```python
from build123d import *

# Parameters (mm, degrees)
F0_W         = 108.091738075
F0_H         = 57.078147307
F1_DEPTH     = 50
F2_T         = -2.5
F3_R         = 1
F4_T1_DEPTH  = 48
F4_T3_DEPTH  = 106.091738075
F4_T5_DEPTH  = 55.078147307
F4_S9_W      = 1
F4_S9_H      = 1
F4_T10_DEPTH = 1
F4_S15_W     = 1
F4_S15_H     = 1
F4_T16_DEPTH = 1
F4_T20_ANGLE = 90
F4_T22_ANGLE = 90
F4_T24_ANGLE = 90
F5_W         = 18.639581278
F5_H         = 12.6642128453
F6_DEPTH     = 25


# Not quite as in the source:
# - a fillet or chamfer that OpenCascade refuses, or shapes differently, is made with other operations: its cross-section is extruded or revolved along the edge and cut away or added


with BuildPart() as f1:
    # F0 (on Top) → F1 (new body)
    with BuildSketch(Plane.XY):
        with Locations((-7.7590625733, 5.3510768339)):
            Rectangle(F0_W, F0_H)
    extrude(amount=F1_DEPTH)

    # F2
    f2_openings = [f1.faces().sort_by_distance(p)[0] for p in [
        (-7.759063, 5.351077, 50),
    ]]
    offset(amount=F2_T, openings=f2_openings)

    # F3
    f3_edges = [f1.edges().sort_by_distance(p)[0] for p in [
        (-7.759063, -23.187997, 50),
        (-61.804932, -23.187997, 25),
        (-7.759063, -20.687997, 50),
        (-59.304932, 5.351077, 50),
        (-61.804932, 5.351077, 50),
        (-7.759063, -23.187997, 0),
        (46.286806, -23.187997, 25),
        (43.786806, 5.351077, 50),
        (46.286806, 5.351077, 50),
        (46.286806, 5.351077, 0),
    ]]
    fillet(f3_edges, radius=F3_R)

    # F4: fillet of radius 1 on 3 edges, made by hand

    # F4_s2 → F4_t1 (cut)
    with BuildSketch(Plane.XY.offset(1)):
        with BuildLine():
            ThreePointArc((45.2868064642, 33.8901504874), (45.9939132454, 33.5972572686), (46.2868064642, 32.8901504874))
            Line((46.2868064642, 32.8901504874), (46.2868064642, 33.8901504874))
            Line((46.2868064642, 33.8901504874), (45.2868064642, 33.8901504874))
        make_face()
        with BuildLine():
            ThreePointArc((-60.8049316108, 33.8901504874), (-61.512038392, 33.5972572686), (-61.8049316108, 32.8901504874))
            Line((-61.8049316108, 32.8901504874), (-61.8049316108, 33.8901504874))
            Line((-61.8049316108, 33.8901504874), (-60.8049316108, 33.8901504874))
        make_face()
    extrude(amount=F4_T1_DEPTH, mode=Mode.SUBTRACT)

    # F4_s4 → F4_t3 (cut)
    with BuildSketch(Plane.YZ.offset(-60.8049316108)):
        with BuildLine():
            ThreePointArc((33.8901504874, 49), (33.5972572686, 49.7071067812), (32.8901504874, 50))
            Line((32.8901504874, 50), (33.8901504874, 50))
            Line((33.8901504874, 50), (33.8901504874, 49))
        make_face()
        with BuildLine():
            ThreePointArc((33.8901504874, 1), (33.5972572686, 0.2928932188), (32.8901504874, 0))
            Line((32.8901504874, 0), (33.8901504874, 0))
            Line((33.8901504874, 0), (33.8901504874, 1))
        make_face()
    extrude(amount=F4_T3_DEPTH, mode=Mode.SUBTRACT)

    # F4_s6 → F4_t5 (cut)
    with BuildSketch(Plane.XZ.offset(-32.8901504874)):
        with BuildLine():
            ThreePointArc((-60.8049316108, 0), (-61.512038392, 0.2928932188), (-61.8049316108, 1))
            Line((-61.8049316108, 1), (-61.8049316108, 0))
            Line((-61.8049316108, 0), (-60.8049316108, 0))
        make_face()
    extrude(amount=F4_T5_DEPTH, mode=Mode.SUBTRACT)


with BuildPart() as f4_tool8:
    # F4_s9 → F4_t10 (new body)
    with BuildSketch(Plane.XY.offset(1)):
        with Locations((-61.3049316108, -22.6879968196)):
            Rectangle(F4_S9_W, F4_S9_H)
    extrude(amount=-F4_T10_DEPTH)

    # F4_s11 → F4_t12 (revolve, cut)
    with BuildSketch(Plane(origin=(-60.8049316108, -22.1879968196, 1), x_dir=(0.7071067812, 0.7071067812, 0), z_dir=(-0.7071067812, 0.7071067812, 0))):
        with BuildLine():
            ThreePointArc((0, -1), (1, 0), (0, 1))
            Line((0, 1), (0, -1))
        make_face()
    revolve(axis=Axis((-60.8049316108, -22.1879968196, 1), (0, 0, -1)), mode=Mode.SUBTRACT)


with BuildPart() as f1_1:
    add(f1.part)

    # F4_t7: cut F4_tool8
    add(f4_tool8.part, mode=Mode.SUBTRACT)


with BuildPart() as f4_tool14:
    # F4_s15 → F4_t16 (new body)
    with BuildSketch(Plane.XZ.offset(-32.8901504874)):
        with Locations((-61.3049316108, 0.5)):
            Rectangle(F4_S15_W, F4_S15_H)
    extrude(amount=-F4_T16_DEPTH)

    # F4_s17 → F4_t18 (revolve, cut)
    with BuildSketch(Plane(origin=(-60.8049316108, 32.8901504874, 1), x_dir=(0.7071067812, 0, 0.7071067812), z_dir=(-0.7071067812, 0, 0.7071067812))):
        with BuildLine():
            ThreePointArc((0, -1), (1, 0), (0, 1))
            Line((0, 1), (0, -1))
        make_face()
    revolve(axis=Axis((-60.8049316108, 32.8901504874, 1), (0, 1, 0)), mode=Mode.SUBTRACT)


with BuildPart() as f1_2:
    add(f1_1.part)

    # F4_t13: cut F4_tool14
    add(f4_tool14.part, mode=Mode.SUBTRACT)

    # F4_s19 → F4_t20 (revolve, cut)
    with BuildSketch(Plane.XY.offset(49)):
        with BuildLine():
            ThreePointArc((45.2868064642, 33.8901504874), (45.9939132454, 33.5972572686), (46.2868064642, 32.8901504874))
            Line((46.2868064642, 32.8901504874), (46.2868064642, 33.8901504874))
            Line((46.2868064642, 33.8901504874), (45.2868064642, 33.8901504874))
        make_face()
    revolve(axis=Axis((45.2868064642, 33.8901504874, 49), (0, -1, 0)), revolution_arc=F4_T20_ANGLE, mode=Mode.SUBTRACT)

    # F4_s21 → F4_t22 (revolve, cut)
    with BuildSketch(Plane.XY.offset(49)):
        with BuildLine():
            ThreePointArc((-60.8049316108, 33.8901504874), (-61.512038392, 33.5972572686), (-61.8049316108, 32.8901504874))
            Line((-61.8049316108, 32.8901504874), (-61.8049316108, 33.8901504874))
            Line((-61.8049316108, 33.8901504874), (-60.8049316108, 33.8901504874))
        make_face()
    revolve(axis=Axis((-60.8049316108, 33.8901504874, 49), (0, 1, 0)), revolution_arc=F4_T22_ANGLE, mode=Mode.SUBTRACT)

    # F4_s23 → F4_t24 (revolve, cut)
    with BuildSketch(Plane.XY.offset(1)):
        with BuildLine():
            ThreePointArc((45.2868064642, 33.8901504874), (45.9939132454, 33.5972572686), (46.2868064642, 32.8901504874))
            Line((46.2868064642, 32.8901504874), (46.2868064642, 33.8901504874))
            Line((46.2868064642, 33.8901504874), (45.2868064642, 33.8901504874))
        make_face()
    revolve(axis=Axis((45.2868064642, 33.8901504874, 1), (0, 1, 0)), revolution_arc=F4_T24_ANGLE, mode=Mode.SUBTRACT)

    # F5 (on face) → F6 (cut)
    with BuildSketch(Plane.YZ.offset(46.2868064642)):
        with Locations((9.319790639, 18.1044735946)):
            Rectangle(F5_W, F5_H)
    extrude(amount=-F6_DEPTH, mode=Mode.SUBTRACT)


solid = f1_2.part
```
Work out the finished part from the listing and answer in its coordinate system (mm). A direction names the side the tool comes from. Coordinates: 2 decimals unless noted, no trailing zeros. Loops run counter-clockwise (first coordinate to the right, second up) from the corner with the lowest first, then second, coordinate; pieces in that order, holes last. Notation, with made-up numbers: M 33.5,-3 L 92.5,-3 A21 ccw 92.5,24 Z; hole C 8,17 d8. An arc over 180 degrees is marked long. Use CSV: the item, a comma, the result in double quotes. Start each with the question number.
(1) Find section B-B, the plane x = 8. Give the vertices of the cut face in (y, z).
(2) Given pin 1 Ø15.5 at (x, y) = (-10.5, 9) entering from +Z, flat-ended and moving along its own axis, determine where the tip first touches the part or whether it passes through.
(3) Find section A-A, the plane y = -15. Give the vertices of the cut face in (x, z).
(4) Find section C-C, the plane z = 4.5. Give the vertices of the cut face in (x, y).
(5) Find section D-D, the plane z = 21. Give the vertices of the cut face in (x, y).
(6) For faces 1 (the face through (45, 0, 18)), 2 (the face through (46.287, 5, 25)), 3 (the face through (-8, 31.39, 26)), determine the directions among +Z, -Z, +X, -X, +Y, -Y from which every point of the face is accessible in a straight line to the end or side of a thin tool.
(7) Consider line 1 (Y direction, x = 39.5, z = 45.5); line 2 (X direction, y = -12, z = 34); line 3 (Z direction, x = 12.5, y = 26). Determine where each line is inside the solid, lowest interval first.
(8) For a pull along X with two mould halves and no side action, classify faces 4 (the face through (-61.805, 5, 25)), 5 (the face through (-59.305, 5, 25)), 6 (the face through (45, 9, 24.437)) as +X half, -X half, draft (parallel to the pull), parting line (faces both ways), or undercut.
Recorded:
1,outline,"M -23.19,1 A1 ccw -22.19,0 L 32.89,0 A1 ccw 33.89,1 L 33.89,49 A1 ccw 32.89,50 L 31.39,50 L 31.39,2.5 L -20.69,2.5 L -20.69,49 A1 ccw -21.69,50 L -22.19,50 A1 ccw -23.19,49 Z"
2,pin 1,"stops at z = 2.5"
3,outline,"M -61.8,1 A1 ccw -60.8,0 L 45.29,0 A1 ccw 46.29,1 L 46.29,49 A1 ccw 45.29,50 L 44.79,50 A1 ccw 43.79,49 L 43.79,2.5 L -59.3,2.5 L -59.3,49 A1 ccw -60.3,50 L -60.8,50 A1 ccw -61.8,49 Z"
4,outline,"M -61.8,-22.19 A1 ccw -60.8,-23.19 L 45.29,-23.19 A1 ccw 46.29,-22.19 L 46.29,32.89 A1 ccw 45.29,33.89 L -60.8,33.89 A1 ccw -61.8,32.89 Z; hole M -59.3,-20.69 L 43.79,-20.69 L 43.79,31.39 L -59.3,31.39 Z"
5,outline,"M -61.8,-22.19 A1 ccw -60.8,-23.19 L 45.29,-23.19 A1 ccw 46.29,-22.19 L 46.29,0 L 43.79,0 L 43.79,-20.69 L -59.3,-20.69 L -59.3,31.39 L 43.79,31.39 L 43.79,18.64 L 46.29,18.64 L 46.29,32.89 A1 ccw 45.29,33.89 L -60.8,33.89 A1 ccw -61.8,32.89 Z"
6,face 1,"+X"
6,face 2,"+Z, -Z, +X, +Y, -Y"
6,face 3,"+Z"
7,line 1,"y = -23.19 to -20.69, 31.39 to 33.89"
7,line 2,"x = -61.8 to -59.3, 43.79 to 46.29"
7,line 3,"z = 0 to 2.5"
8,face 4,"-X half"
8,face 5,"undercut"
8,face 6,"draft"
